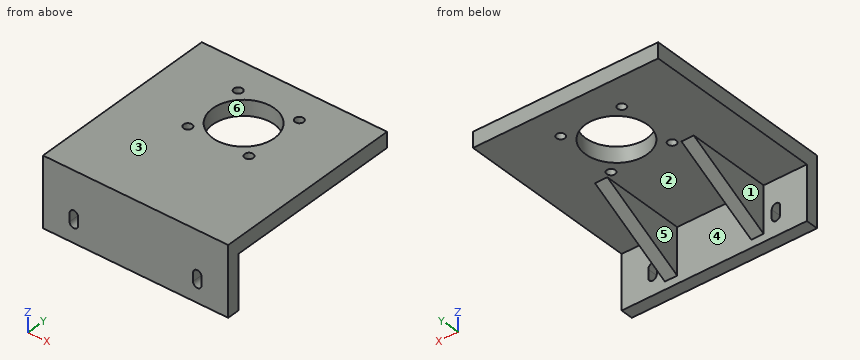
```python
from build123d import *

# Parameters (mm, degrees)
SKETCH_1_W          = 120
SKETCH_1_H          = 125
SKETCH_1_R          = 20
SKETCH_1_R_2        = 2.75
EXTRUDE_1_DEPTH     = 10
SKETCH_2_W          = 120
SKETCH_2_H          = 35
EXTRUDE_3_DEPTH     = 8
EXTRUDE_4_DEPTH     = 32
CUT_EXTRUDE_1_DEPTH = 24


with BuildPart() as part:
    # 草图1 → 凸台-拉伸1 (new body)
    with BuildSketch(Plane.XY):
        with Locations((0, 62.5)):
            Rectangle(SKETCH_1_W, SKETCH_1_H)
        with Locations((0, 85)):
            Circle(SKETCH_1_R, mode=Mode.SUBTRACT)
        with Locations((19.798989873, 104.798989873)):
            Circle(SKETCH_1_R_2, mode=Mode.SUBTRACT)
        with Locations((-19.798989873, 104.798989873)):
            Circle(SKETCH_1_R_2, mode=Mode.SUBTRACT)
        with Locations((-19.798989873, 65.201010127)):
            Circle(SKETCH_1_R_2, mode=Mode.SUBTRACT)
        with Locations((19.798989873, 65.201010127)):
            Circle(SKETCH_1_R_2, mode=Mode.SUBTRACT)
    extrude(amount=-EXTRUDE_1_DEPTH)

    # 草图2 → 凸台-拉伸3 (add)
    with BuildSketch(Plane(origin=(0, 0, 0), x_dir=(1, 0, 0), z_dir=(0, 1, 0))):
        with Locations((0, 27.5)):
            Rectangle(SKETCH_2_W, SKETCH_2_H)
        with BuildLine():
            Line((-42.75, 27.5), (-42.75, 33))
            ThreePointArc((-42.75, 33), (-40, 35.75), (-37.25, 33))
            Line((-37.25, 33), (-37.25, 27.5))
            ThreePointArc((-37.25, 27.5), (-40, 24.75), (-42.75, 27.5))
        make_face(mode=Mode.SUBTRACT)
        with BuildLine():
            Line((37.25, 27.5), (37.25, 33))
            ThreePointArc((37.25, 33), (40, 35.75), (42.75, 33))
            Line((42.75, 33), (42.75, 27.5))
            ThreePointArc((42.75, 27.5), (40, 24.75), (37.25, 27.5))
        make_face(mode=Mode.SUBTRACT)
    extrude(amount=EXTRUDE_3_DEPTH)

    # 草图3 → 凸台-拉伸4 (add, symmetric)
    with BuildSketch(Plane(origin=(0, 0, 0), x_dir=(0, 0, -1), z_dir=(1, 0, 0))):
        Polygon((10, 8), (40, 8), (10, 63), align=None)
    extrude(amount=EXTRUDE_4_DEPTH, both=True)

    # 草图4 → 切除-拉伸1 (cut, symmetric)
    with BuildSketch(Plane(origin=(0, 0, 0), x_dir=(0, 0, -1), z_dir=(1, 0, 0))):
        Polygon((10, 8), (40, 8), (10, 63), align=None)
    extrude(amount=CUT_EXTRUDE_1_DEPTH, both=True, mode=Mode.SUBTRACT)


solid = part.part
```
Geometry: final body of the model. Coordinates: model frame, mm. Face numbers are marked on the shaded views. A direction names the side the tool comes from. Round coordinates to 2 decimals unless told otherwise and drop trailing zeros. Loops run counter-clockwise (first coordinate to the right, second up) from the corner with the lowest first, then second, coordinate; pieces in that order, holes last.
Item 1: Contact query for flat-ended pins moving along their axis: P1, Ø7, axis at x = -19.8, y = 65.2, coming from the -Z side; P2, Ø9, axis at y = 39.5, z = -17.5, coming from the -X side; P3, Ø10.5, axis at x = 12.5, z = -27.5, coming from the +Y side; P4, Ø9, axis at y = 42.5, z = -31, coming from the -X side. Output: stop coordinate, or through.
Checked values:
P1: stops at z = -10
P2: stops at x = -32
P3: stops at y = 8
P4: passes through
Item 2: Reachability of the marked faces 1, 2 and 3 from +Z, -Z, +X, -X, +Y, -Y: full face, straight path, thin tool, end or side. Return the list, or none.
Checked values:
face 1: -Z, -X, +Y
face 2: -Z, +Y
face 3: +Z, +X, -X, +Y, -Y
Item 3: Line query: L1, parallel to Y at x = 0, z = -6; L2, parallel to Y at x = 47.5, z = -17.5; L3, parallel to Z at x = -9, y = 10.5. Output: solid intervals per line, ascending.
Checked values:
L1: y = 0 to 65, 105 to 125
L2: y = 0 to 8
L3: z = -10 to 0
Item 4: Section A-A, the plane y = 85. Output: boundary loops of the cut face in (x, z).
Checked values:
outline: (-60, -10) - (-20, -10) - (-20, 0) - (-60, 0) - close; (20, -10) - (60, -10) - (60, 0) - (20, 0) - close
Item 5: Section C-C, the plane z = -13. Output: boundary loops of the cut face in (x, y), plus the area to 3 significant figures.
Checked values:
outline: (-60, 0) - (60, 0) - (60, 8) - (32, 8) - (32, 57.5) - (24, 57.5) - (24, 8) - (-24, 8) - (-24, 57.5) - (-32, 57.5) - (-32, 8) - (-60, 8) - close
area: 1,750 mm2
Item 6: Section D-D, the plane x = 40. Output: boundary loops of the cut face in (y, z), plus the area to 3 significant figures.
Checked values:
outline: (0, -45) - (8, -45) - (8, -35.75) - (0, -35.75) - close; (0, -24.75) - (8, -24.75) - (8, -10) - (125, -10) - (125, 0) - (0, 0) - close
area: 1,440 mm2
Item 7: Mould query, pull axis Y, two halves, no side actions, for the marked faces 4, 5 and 6. Classes: released by +Y, released by -Y, zero draft, split by the parting line, or undercut.
Checked values:
face 4: released by +Y
face 5: zero draft
face 6: undercut
Item 8: Section B-B, the plane x = 0. Output: boundary loops of the cut face in (y, z).
Checked values:
outline: (0, -45) - (8, -45) - (8, -10) - (65, -10) - (65, 0) - (0, 0) - close; (105, -10) - (125, -10) - (125, 0) - (105, 0) - close
